Check sheet for the drawn part. Datum: minimum x, y, z corner. Units: mm. A direction names the side the tool comes from. Coordinates: 2 decimals unless noted, no trailing zeros. Write each loop counter-clockwise with the first axis right and the second up, starting at its lowest first coordinate (ties: lowest second). Pieces come first, ordered by that corner, then holes. Notation, with made-up numbers: M 46.5,-34 L 103.5,-34 A23 ccw 103.5,-18 Z; hole C 79,4 d5. An arc over 180 degrees is marked long. Answer in a Markdown table with one row per item.
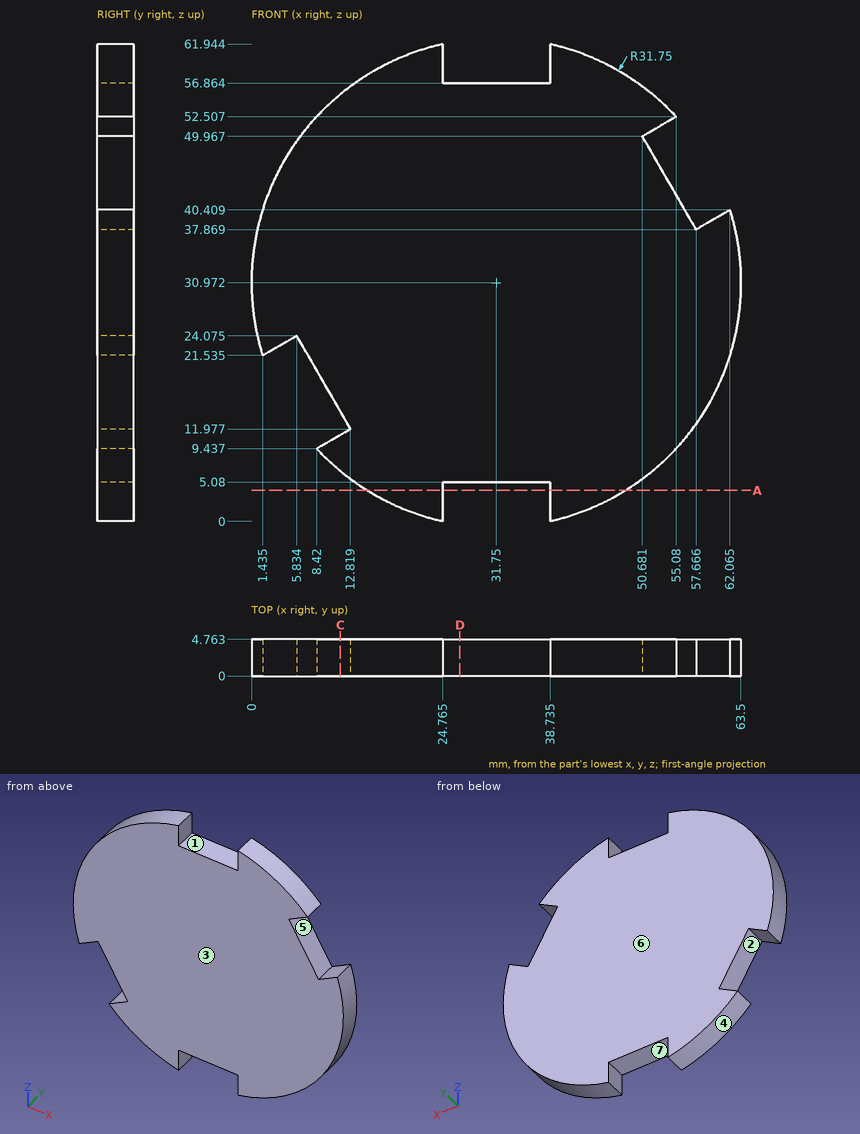
1) Sectioned sample at D-D (x = 27). Record the cut outline in (y, z) (1 decimal).
Response values:
| item | result |
|---|---|
| outline | M 0,5.1 L 4.8,5.1 L 4.8,56.9 L 0,56.9 Z |
2) Depth check by flat-ended pin: pin 1 (1.5 mm diameter, centred on x = 12.5, y = 2, fed in from +Z) (1 decimal); pin 2 (1.4 mm diameter, centred on y = 3, z = 1.5, fed in from +X) (1 decimal); pin 3 (1.4 mm diameter, centred on y = 2.5, z = 2.5, fed in from -X) (1 decimal). Enter the tip coordinate at first touch or a pass-through.
Response values:
| item | result |
|---|---|
| pin 1 | stops at z = 56.8 |
| pin 2 | stops at x = 45.2 |
| pin 3 | stops at x = 16.4 |
3) Tool access check on the marked faces 5, 6 and 7. Record the directions out of +Z, -Z, +X, -X, +Y, -Y that give a thin tool (end or side, any length) a straight path to the whole face; none if there is none.
Response values:
| item | result |
|---|---|
| face 5 | +Y, -Y |
| face 6 | +Z, -Z, +X, -X, +Y |
| face 7 | -Z, +Y, -Y |
4) Thickness scan on L1, parallel to Z at x = 36, y = 2.7 (1 decimal); L2, parallel to X at y = 3.65, z = 52.5 (1 decimal); L3, parallel to X at y = 1.65, z = 5 (1 decimal). Record the ranges inside material, lowest first. Write a range as [from, to].
Response values:
| item | result |
|---|---|
| L1 | z = [5.1, 56.9] |
| L2 | x = [8.4, 55.1] |
| L3 | x = [13.5, 24.8], [38.7, 50] |
5) Sectioned sample at A-A (z = 4). Record the cut outline in (x, y) (1 decimal).
Response values:
| item | result |
|---|---|
| outline | M 15,0 L 24.8,0 L 24.8,4.8 L 15,4.8 Z; M 38.7,0 L 48.5,0 L 48.5,4.8 L 38.7,4.8 Z |
6) Release check for a two-part mould opening along Z. For the marked faces 1, 2, 3 and 4 record: +Z half, -Z half, draft (parallel to the pull), parting line (faces both ways), or undercut.
Response values:
| item | result |
|---|---|
| face 1 | +Z half |
| face 2 | undercut |
| face 3 | draft |
| face 4 | -Z half |
7) Sectioned sample at C-C (x = 11.5). Record the cut outline in (y, z) (1 decimal).
Response values:
| item | result |
|---|---|
| outline | M 0,6.5 L 4.8,6.5 L 4.8,11.2 L 0,11.2 Z; M 0,14.3 L 4.8,14.3 L 4.8,55.4 L 0,55.4 Z |
